Read the model definition and answer for the solid it produces. Units are mm, in the model's axes. Coordinates: 2 decimals unless noted, no trailing zeros. Loops run counter-clockwise (first coordinate to the right, second up) from the corner with the lowest first, then second, coordinate; pieces in that order, holes last. Notation, with made-up numbers: M 29.5,23 L 37.5,23 A27 cw 37.5,62 Z; hole C -14,4.25 d6. An arc over 180 degrees is marked long. One line per item, written item: value. Start each with the question number.
1. Consider probe 1 along Y at (x, z) = (132.5, 0.7); probe 2 along Y at (x, z) = (156.5, 2.35) (3 decimals); probe 3 along X at (y, z) = (9, 1.9). Determine where each line is inside the solid, lowest interval first.
2. Flat-ended cylindrical pins translate along their axes: pin 1 (4 mm diameter, centred on x = 132.715, y = 10.795, fed in from +Z); pin 2 (1 mm diameter, centred on y = 5.5, z = 1.5, fed in from -X); pin 3 (5.5 mm diameter, centred on x = 179.959, y = 10.795, fed in from -Z). Find the tip coordinate at first contact, or state that the pin passes through.
3. Determine the mould class of faces 1 (the face through (182.35, 21.27, 1.29)), 2 (the face through (148, 27, 0)), 3 (the face through (1.81, 1.91, 1.29)), 4 (the face through (182.35, 11.11, 1.29)) for opening direction X: +X half, -X half, draft (parallel to the pull), parting line (faces both ways), or undercut.
4. The part is cut by section A-A (x = 140). Write down the section's boundary in (y, z) (3 decimals).
5. The part is cut by section B-B (z = 2.1). State how many separate pieces and enclosed holes the cut face has, then the cut area to 3 significant figures.
Solid Edge part; units mm, degrees
sketch "Sketch1" plane through (0, 0, 0) normal (0, 0, 1) x (1, 0, 0)
  line L0 (0, 0) -> (0, 31.75)
  line L1 (0, 31.75) -> (292.1, 31.75)
  line L2 (292.1, 31.75) -> (292.1, 0)
  line L3 (292.1, 0) -> (0, 0)
  dimension "D1" = 292.1
extrude "Protrusion1" add sketch "Sketch1" along normal blind 2.54
hole "Hole_1" at (287.3375, 15.875, 2.54) direction (0, 0, -1) diameter 5.5626 end up to next
hole "Hole1" at (4.7625, 15.875, 2.54) direction (0, 0, -1) diameter 5.5626 end up to next
fillet "Round_1" radius 6.35 4 edges at (0, 0, 1.27) (0, 31.75, 1.27) (292.1, 31.75, 1.27) (292.1, 0, 1.27)
sketch "Sketch2" plane through (146.05, 25.4, 2.54) normal (0, 0, 1) x (1, 0, 0)
  line L0 (-9.779, 0.635) -> (-9.779, -19.685)
  line L1 (-9.779, -19.685) -> (30.353, -19.685)
  line L2 (30.353, -19.685) -> (30.353, 0.635)
  line L3 (30.353, 0.635) -> (-9.779, 0.635)
  dimension "D1" = 30.353
  dimension "D2" = 9.779
extrude "Cutout1" cut sketch "Sketch2" against normal through all
hole "Hole2" at (179.959, 20.955, 2.54) direction (0, 0, -1) diameter 4.826 end through all
hole "Hole3" at (179.959, 10.795, 2.54) direction (0, 0, -1) diameter 4.826 end through all
hole "Hole4" at (132.715, 10.795, 2.54) direction (0, 0, -1) diameter 4.826 end through all
hole "Hole5" at (132.715, 20.955, 2.54) direction (0, 0, -1) diameter 4.826 end through all
properties part number "SR-04"
Answer block:
1. probe 1: y = 0 to 8.39, 13.2 to 18.55, 23.36 to 31.75
1. probe 2: y = 0 to 5.715, 26.035 to 31.75
1. probe 3: x = 0 to 131.1, 134.33 to 136.27, 176.4 to 178.35, 181.57 to 292.1
2. pin 1: passes through
2. pin 2: stops at x = 0.01
2. pin 3: stops at z = 0
3. face 1: undercut
3. face 2: draft
3. face 3: -X half
3. face 4: undercut
4. outline: M 0,0 L 5.715,0 L 5.715,2.54 L 0,2.54 Z; M 26.035,0 L 31.75,0 L 31.75,2.54 L 26.035,2.54 Z
5. separate pieces: 1
5. enclosed holes: 7
5. area: 8,300 mm2
